```python
from build123d import *

# Parameters (mm, degrees)
SKETCH_R        = 63.794686
PAD_DEPTH       = 31
POCKET_DEPTH    = 10
POCKET001_DEPTH = 23
SKETCH003_R     = 5.75
POCKET002_DEPTH = 31.001


with BuildPart() as part:
    # Sketch → Pad (new body)
    with BuildSketch(Plane.XY):
        with Locations((5.42, -16.5)):
            Circle(SKETCH_R)
    extrude(amount=PAD_DEPTH)

    # Sketch001 (on Face6 of Pad) → Pocket (cut)
    with BuildSketch(Plane.XY.offset(31)):
        Polygon((-18.08, 0.5), (51.5, 0.5), (51.5, -2.802), (101.5, -2.802), (101.5, -12.692), (51.5, -12.692), (51.5, -31.25), (101.5, -31.25), (101.5, -44.2261), (51.5, -44.2261), (51.5, -53.84), (-18.08, -53.84), align=None)
    extrude(amount=-POCKET_DEPTH, mode=Mode.SUBTRACT)

    # Sketch002 (on Face7 of Pocket) → Pocket001 (cut)
    with BuildSketch(Plane.XY.offset(31)):
        with BuildLine():
            ThreePointArc((-5.83, -16.5), (5.42, -27.75), (16.67, -16.5))
            Line((16.67, -16.5), (16.67, 0))
            Line((16.67, 10), (16.67, 0))
            Line((-5.83, 10), (16.67, 10))
            Line((-5.83, 0), (-5.83, 10))
            Line((-5.83, -16.5), (-5.83, 0))
        make_face()
    extrude(amount=-POCKET001_DEPTH, mode=Mode.SUBTRACT)

    # Sketch003 (on Face7 of Pocket001) → Pocket002 (cut, through all)
    with BuildSketch(Plane.XY.offset(31)):
        with Locations((5.42, -16.5)):
            Circle(SKETCH003_R)
    extrude(amount=-POCKET002_DEPTH, mode=Mode.SUBTRACT)


solid = part.part
```
The model under review builds one solid part; all positions refer to its coordinate system, in mm. A direction names the side the tool comes from. Give positions to 0.01 mm unless a question says otherwise; leave off trailing zeros. Write each loop counter-clockwise with the first axis right and the second up, starting at its lowest first coordinate (ties: lowest second). Pieces come first, ordered by that corner, then holes.
(1) Consider section D-D, the plane y = -37.5. Give the boundary of the cut face in (x, z).
(2) Tool access review of faces 4 (the flat face through (5, -4, 8)), 5 (the flat face through (60, -12.692, 26)), 6 (the flat face through (60, -22, 31)): name each direction out of +Z, -Z, +X, -X, +Y, -Y from which nothing blocks a thin tool from reaching the whole face with its end or side.
(3) To check wall thickness, follow L1, parallel to Y at x = 5.42, z = 6; L2, parallel to Z at x = 44.5, y = -43.5; L3, parallel to X at y = 5, z = 19.5. State the ranges of each line that lie inside material, in increasing order.
(4) For P1, Ø4, axis at x = 4, z = 8.5, coming from the -Y side; P2, Ø5, axis at y = -21, z = 26, coming from the -X side; P3, Ø3, axis at x = -14, z = 27, coming from the -Y side, all flat-tipped, find the tip position at first contact; note any pin that passes through.
(5) Consider section A-A, the plane x = 5.42. Give the boundary of the cut face in (y, z), and give its area (3 significant figures).
(6) Consider section C-C, the plane x = 33. Give the boundary of the cut face in (y, z), and give its area (3 significant figures).
(7) Consider section B-B, the plane y = 3. Give the boundary of the cut face in (x, z).
(8) The part is to be moulded in two halves that separate along X. For faces 1 (the flat face through (51.5, -49, 26)), 2 (the cylindrical face through (-58.313, -13.695, 15.283)), 3 (the flat face through (59, -2.802, 26)), say which applies: released by +X, released by -X, zero draft, split by the parting line, or undercut.
Returned:
1. outline: (-54.82, 0) - (65.66, 0) - (65.66, 21) - (-18.08, 21) - (-18.08, 31) - (-54.82, 31) - close
2. face 4: +Z
2. face 5: +Z, +X
2. face 6: +Z, +X, -X, +Y, -Y
3. L1: y = -80.29 to -22.25, -10.75 to 47.29
3. L2: z = 0 to 21
3. L3: x = -54.64 to -5.83, 16.67 to 65.48
4. P1: stops at y = -80.29
4. P2: stops at x = -58.34
4. P3: stops at y = -77.73
5. outline: (-80.29, 0) - (-22.25, 0) - (-22.25, 8) - (-27.75, 8) - (-27.75, 21) - (-53.84, 21) - (-53.84, 31) - (-80.29, 31) - close; (-10.75, 0) - (47.29, 0) - (47.29, 31) - (10, 31) - (10, 8) - (-10.75, 8) - close
5. area: 2,730 mm2
6. outline: (-74.02, 0) - (41.02, 0) - (41.02, 31) - (0.5, 31) - (0.5, 21) - (-53.84, 21) - (-53.84, 31) - (-74.02, 31) - close
6. area: 3,020 mm2
7. outline: (-55.32, 0) - (66.16, 0) - (66.16, 31) - (16.67, 31) - (16.67, 8) - (-5.83, 8) - (-5.83, 31) - (-55.32, 31) - close
8. face 1: undercut
8. face 2: split by the parting line
8. face 3: zero draft
